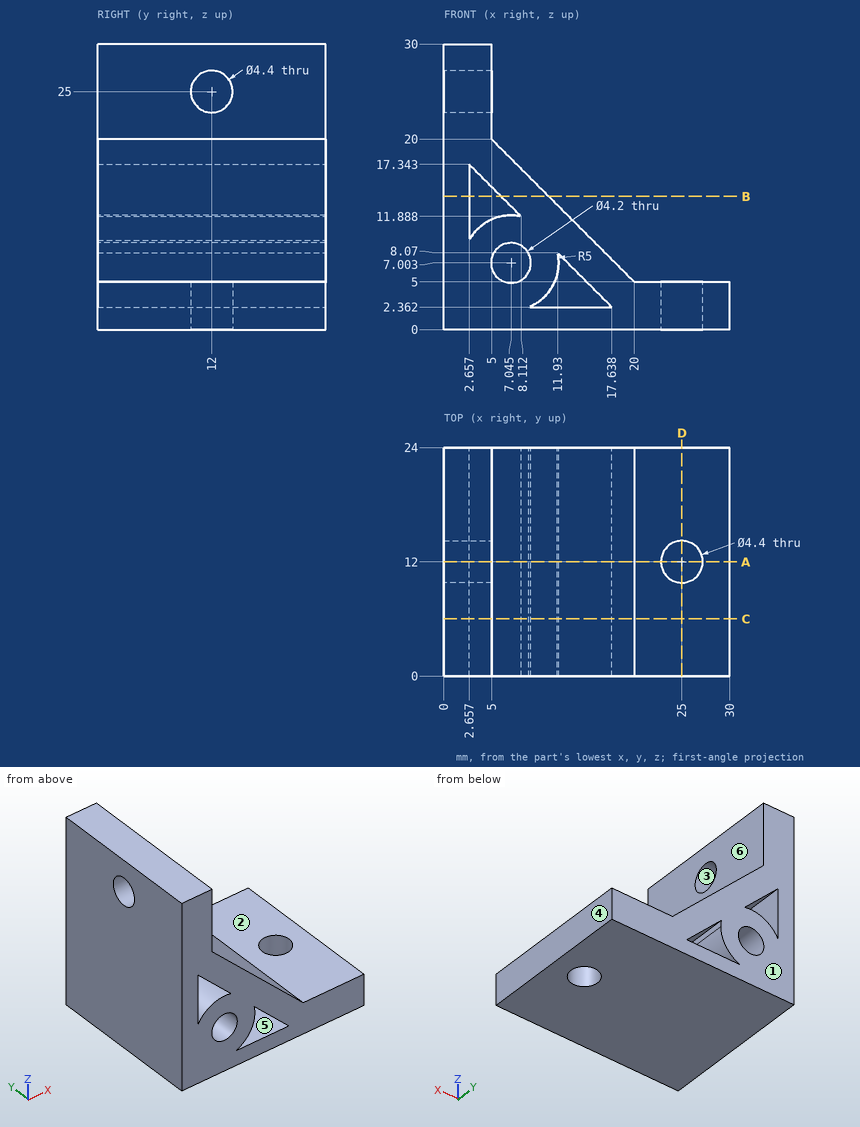
Here's the drawing with two shaded views (mm, measured from the low corner). I have some questions. A direction names the side the tool comes from. Coordinates: 2 decimals unless noted, no trailing zeros. Order: outer loops, then holes, each group sorted by start corner. A loop starts at its lowest first (then second) coordinate and runs counter-clockwise, first axis right, second up.
Item 1: I need wall thicknesses on probe 1 along Y at (x, z) = (25, 3.6); probe 2 along Z at (x, y) = (7, 11.5) (1 decimal); probe 3 along Z at (x, y) = (2.45, 12). Which ranges of each line are inside material? Lowest first, please.
Response values:
probe 1: y = 0 to 9.8, 14.2 to 24
probe 2: z = 0 to 4.9, 9.1 to 12, 13 to 18
probe 3: z = 0 to 22.8, 27.2 to 30
Item 2: If we section it at C-C, the plane y = 6: List the corners of the cut face in (x, z) for me (1 decimal).
Response values:
outline: (0, 0) - (30, 0) - (30, 5) - (20, 5) - (5, 20) - (5, 30) - (0, 30) - close; hole (2.7, 9.4) arc R5 cw to (8.1, 11.9) - (2.7, 17.3) - close; hole circle Ø4.2 at (7, 7); hole (8.9, 2.4) - (17.6, 2.4) - (11.9, 8.1) arc R5 cw to start
Item 3: I'm going to push flat-ended pins straight in: pin 1 Ø9.5 at (x, y) = (12.5, 8) entering from +Z; pin 2 Ø4 at (y, z) = (20.5, 17.5) entering from +X; pin 3 Ø2.5 at (y, z) = (17, 12) entering from +X. Where does each tip first touch, or does it pass through?
Response values:
pin 1: stops at z = 17.25
pin 2: stops at x = 9.5
pin 3: stops at x = 14.25
Item 4: If we section it at A-A, the plane y = 12: List the corners of the cut face in (x, z) for me (1 decimal).
Response values:
outline: (0, 0) - (22.8, 0) - (22.8, 5) - (20, 5) - (5, 20) - (5, 22.8) - (0, 22.8) - close; (0, 27.2) - (5, 27.2) - (5, 30) - (0, 30) - close; (27.2, 0) - (30, 0) - (30, 5) - (27.2, 5) - close; hole (2.7, 9.4) arc R5 cw to (8.1, 11.9) - (2.7, 17.3) - close; hole circle Ø4.2 at (7, 7); hole (8.9, 2.4) - (17.6, 2.4) - (11.9, 8.1) arc R5 cw to start
Item 5: Which directions (+Z, -Z, +X, -X, +Y, -Y) give clear straight access to the entire face, cutting with the end or side of a thin tool? Please do the marked faces 4, 5 and 6.
Response values:
face 4: +Z, -Z, +X, +Y, -Y
face 5: +Y, -Y
face 6: +Z, +X, +Y, -Y
Item 6: Thinking about a two-plate mould opening in Z: for the marked faces 1, 2 and 3, which applies, pulls with the +Z half, pulls with the -Z half, needs draft (parallel to the pull), parting line crosses it, or undercut?
Response values:
face 1: needs draft
face 2: pulls with the +Z half
face 3: undercut
Item 7: If we section it at B-B, the plane z = 14: List the corners of the cut face in (x, y) for me, then the cut area to 3 significant figures.
Response values:
outline: (0, 0) - (2.66, 0) - (2.66, 24) - (0, 24) - close; (6, 0) - (11, 0) - (11, 24) - (6, 24) - close
area: 184 mm2
Item 8: If we section it at D-D, the plane x = 25: List the corners of the cut face in (y, z) for me, then the cut area to 3 significant figures.
Response values:
outline: (0, 0) - (9.8, 0) - (9.8, 5) - (0, 5) - close; (14.2, 0) - (24, 0) - (24, 5) - (14.2, 5) - close
area: 98.0 mm2
